Part model, mm, in its own coordinate system. Face numbers are marked on the shaded views. A direction names the side the tool comes from. Coordinates: 2 decimals unless noted, no trailing zeros. Write each loop counter-clockwise with the first axis right and the second up, starting at its lowest first coordinate (ties: lowest second). Pieces come first, ordered by that corner, then holes. Notation, with made-up numbers: (-23, -1) -> (28, -1) arc R28 ccw to (28, 37) -> close; hole circle Ø3 at (49.25, -25.5). An arc over 180 degrees is marked (long way). Write item = value, one per line.
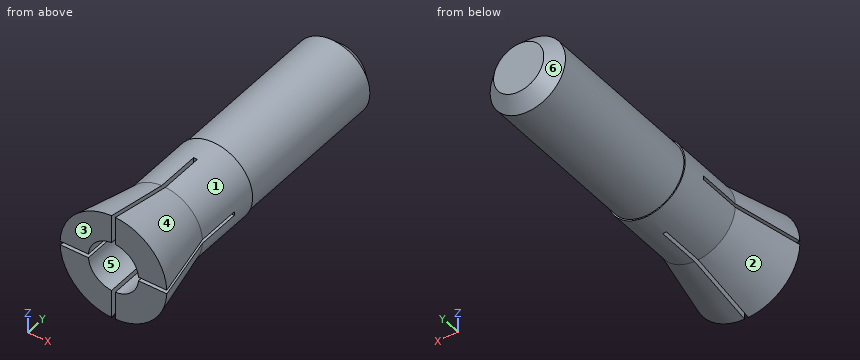
Autodesk Inventor part; units mm, degrees
ref_plane "YZ Plane" through (0, 0, 0) normal (1, 0, 0) x (0, 1, 0)
ref_plane "XZ Plane" through (0, 0, 0) normal (0, 1, 0) x (-1, 0, 0)
ref_plane "XY Plane" through (0, 0, 0) normal (0, 0, 1) x (1, 0, 0)
sketch "Sketch1" plane through (0, 0, 0) normal (0, 0, 1) x (1, 0, 0)
  line L0 (0, 0) -> (-4.25, 0) construction
  line L1 (-4.25, 0) -> (-4.25, 5.5) construction
  line L2 (-4.25, 5.5) -> (0, 5.5) construction
  line L3 (0, 5.5) -> (0, 0) construction
  line L4 (0, 5.5) -> (-3.1, 5.5) construction
  line L5 (-3.1, 5.5) -> (-3.1, 11) construction
  line L6 (-3.1, 11) -> (0, 11) construction
  line L7 (0, 11) -> (0, 5.5) construction
  line L8 (0, 0) -> (-4.25, 0)
  line L9 (-4.25, 0) -> (-3.1, 5.5)
  line L10 (-3.1, 5.5) -> (-3.1, 11)
  line L11 (-3.1, 11) -> (0, 11)
  line L12 (0, 11) -> (0, 0)
  dimension "d0" = 5.5
  dimension "d1" = 4.25
  dimension "d2" = 5.5
  dimension "d3" = 3.1
revolve "Revolution1" add sketch "Sketch1" angle 360 about axis through (0, 11, 0) along (0, -1, 0)
sketch "Sketch2" plane through (0, 11, 0) normal (0, 1, 0) x (1, 0, 0)
  circle A0 centre (0, 0) radius 3
  circle A1 centre (0, 0) radius 3.1 construction
  dimension "d5" = 6
extrude "Extrusion1" add sketch "Sketch2" along normal blind 14
thread "Thread1"
chamfer "Chamfer1" distance 1 angle 45 1 edges at (-3, 25, 0)
sketch "Sketch3" plane through (0, 0, 0) normal (0, -1, 0) x (1, 0, 0)
  point P0 (0, 0)
  point P1 (0, 0)
hole "Hole1" at (0, 0, 0) direction (0, 1, 0) diameter 4 depth 11 tip angle 118
sketch "Sketch4" plane through (0, 0, 0) normal (1, 0, 0) x (0, 1, 0)
  line L0 (0, -4.25) -> (0, 4.25)
  line L1 (0, 4.25) -> (9, 4.25)
  line L2 (9, 4.25) -> (9, -4.25)
  line L3 (9, -4.25) -> (0, -4.25)
  line L4 (0, -4.25) -> (0, 4.25)
  point P0 (0, 0)
  dimension "d20" = 9
extrude "Extrusion2" cut sketch "Sketch4" along normal mid plane 0.3
sketch "Sketch5" plane through (0, 0, 0) normal (0, 0, 1) x (1, 0, 0)
  line L0 (4.25, 0) -> (3.1, 5.5)
  line L1 (4.25, 0) -> (-4.25, 0)
  line L2 (-4.25, 0) -> (-4.25, 9)
  line L3 (-4.25, 9) -> (4.25, 9)
  line L4 (4.25, 9) -> (4.25, 0)
  line L5 (0.15, 0) -> (0.15, 5.5) construction
  line L6 (0.15, 5.5) -> (0.15, 5.5) construction
  line L7 (0.15, 5.5) -> (0.15, 0) construction
  line L8 (0.15, 0) -> (0.15, 0) construction
  line L9 (-0.15, 5.5) -> (-0.15, 0) construction
  line L10 (-0.15, 0) -> (-0.15, 0) construction
  line L11 (-0.15, 0) -> (-0.15, 5.5) construction
  line L12 (-0.15, 5.5) -> (-0.15, 5.5) construction
  line L13 (-4.25, 0) -> (-3.1, 5.5) construction
  line L14 (-0.15, 0) -> (-4.25, 0) construction
  point P0 (0, 0)
  dimension "d23" = 9
extrude "Extrusion3" cut sketch "Sketch5" along normal mid plane 0.3
properties part number "collet_screw" material "Aluminum 6061"
Q1. Saw through at B-B on y = 16.75. Give the cut face in (x, z).
Model answer:
outline = circle Ø6 at (0, 0)
Q2. Saw through at A-A on y = 6. Give the cut face in (x, z), and give its area (3 significant figures).
Model answer:
outline = (-3.1, -0.15) arc R3.1 ccw to (-0.15, -3.1) -> (-0.15, -1.99) arc R2 cw to (-1.99, -0.15) -> close; (-3.1, 0.15) -> (-1.99, 0.15) arc R2 cw to (-0.15, 1.99) -> (-0.15, 3.1) arc R3.1 ccw to start; (0.15, -3.1) arc R3.1 ccw to (3.1, -0.15) -> (1.99, -0.15) arc R2 cw to (0.15, -1.99) -> close; (0.15, 1.99) arc R2 cw to (1.99, 0.15) -> (3.1, 0.15) arc R3.1 ccw to (0.15, 3.1) -> close
area = 16.3 mm²
Q3. Which spindle directions (+Z, -Z, +X, -X, +Y, -Y) get a long thin tool onto all of the face, cutting with end or side? Do the marked faces 1 and 2. Say none if no direction does.
Model answer:
face_1 = +Y
face_2 = -Z, -X, +Y
Q4. Pin check, flat tips, straight feed: pin 1 (2.5 mm diameter, centred on x = -2.5, y = 5, fed in from +Z); pin 2 (1.5 mm diameter, centred on x = -1, y = 11.5, fed in from +Z); pin 3 (1.1 mm diameter, centred on y = 5, z = -3, fed in from +X). Stop position of each tip, or through.
Model answer:
pin_1 = 3.02
pin_2 = 3.07
pin_3 = 2.09
Q5. Mould opens along Z. For the marked faces 3, 4, 5 and 6 say: released by +Z, released by -Z, zero draft, split by the parting line, or undercut.
Model answer:
face_3 = zero draft
face_4 = released by +Z
face_5 = undercut
face_6 = split by the parting line
Q6. Probe line 1 (X direction, y = 2, z = -1.5); line 2 (Z direction, x = 2.5, y = 5.25); line 3 (Z direction, x = -0.25, y = 5.5). List the from-to ranges inside material, lowest first. Write a range as from..to.
Model answer:
line_1 = -3.53..-1.32, 1.32..3.53
line_2 = -1.92..-0.15, 0.15..1.92
line_3 = -3.09..-1.98, 1.98..3.09
